Input: part model. Units: mm. Frame: model coordinates. Coordinates: 2 decimals unless noted, no trailing zeros. Loops run counter-clockwise (first coordinate to the right, second up) from the corner with the lowest first, then second, coordinate; pieces in that order, holes last.
(1) Section A-A, the plane y = -54.5. Return loops of the section in (x, z), then the cut area to 3 significant figures.
(2) Line query: L1, parallel to Z at x = 4, y = -49; L2, parallel to Z at x = 27.5, y = -34.5; L3, parallel to Z at x = 63, y = -6. Output: solid intervals per line, ascending.
(3) Contact query for flat-ended pins moving along their axis: P1, Ø5, axis at x = 10.5, y = -32.5, coming from the +Z side; P2, Ø12, axis at x = 9, y = -52.5, coming from the +Z side; P3, Ø4, axis at x = -63, y = -18, coming from the -Z side. Output: stop coordinate, or through.
(4) Section B-B, the plane x = 70. Return loops of the section in (y, z), then the cut area to 3 significant figures.
(5) Mould query, pull axis Z, two halves, no side actions, for faces 1 (the face through (-11.012, -37.567, -49.592)), 2 (the face through (-1, 0, 774)). Classes: released by +Z, released by -Z, zero draft, split by the parting line, or undercut.
(6) Section C-C, the plane x = -87. Return loops of the section in (y, z), then the cut area to 3 significant figures.
```python
from build123d import *

# Parameters (mm, degrees)
F0_R     = 50.8
F1_DEPTH = 76.2


with BuildPart() as f1:
    # F0 (on Front) → F1 (new body)
    with BuildSketch(Plane.XZ):
        with BuildLine():
            Line((-101.6, 1524), (-101.6, 0))
            ThreePointArc((-101.6, 0), (-71.842049, -71.842049), (0, -101.6))
            ThreePointArc((0, -101.6), (71.842049, -71.842049), (101.6, 0))
            Line((101.6, 0), (101.6, 1524))
            ThreePointArc((101.6, 1524), (71.842049, 1595.842049), (0, 1625.6))
            ThreePointArc((0, 1625.6), (-71.842049, 1595.842049), (-101.6, 1524))
        make_face()
        Circle(F0_R, mode=Mode.SUBTRACT)
        with Locations((0, 1524)):
            Circle(F0_R, mode=Mode.SUBTRACT)
    extrude(amount=F1_DEPTH)


solid = f1.part
```
Report:
1. outline: (-101.6, 0) arc R101.6 ccw to (101.6, 0) - (101.6, 1524) arc R101.6 ccw to (-101.6, 1524) - close; hole circle Ø101.6 at (0, 0); hole circle Ø101.6 at (0, 1524)
1. area: 326,000 mm2
2. L1: z = -101.52 to -50.64, 50.64 to 1473.36, 1574.64 to 1625.52
2. L2: z = -97.81 to -42.71, 42.71 to 1481.29, 1566.71 to 1621.81
2. L3: z = -79.71 to 1603.71
3. P1: stops at z = 1625.28
3. P2: stops at z = 1625.56
3. P3: stops at z = -81.25
4. outline: (-76.2, -73.64) - (0, -73.64) - (0, 1597.64) - (-76.2, 1597.64) - close
4. area: 127,000 mm2
5. face 1: undercut
5. face 2: zero draft
6. outline: (-76.2, -52.47) - (0, -52.47) - (0, 1576.47) - (-76.2, 1576.47) - close
6. area: 124,000 mm2
